Could you check a few things on this model? Use its own coordinates, in mm. Face numbers are marked on the shaded views. Give positions to 0.01 mm unless a question says otherwise; leave off trailing zeros. Write each loop counter-clockwise with the first axis right and the second up, starting at its lowest first coordinate (ties: lowest second). Pieces come first, ordered by that corner, then holes. Notation, with made-up numbers: (79.5, -35) - (116.5, -35) arc R30 ccw to (116.5, 2) - close; hole circle Ø2 at (-18, 46). An arc over 180 degrees is marked (long way). Answer in a Markdown table with one row per item.
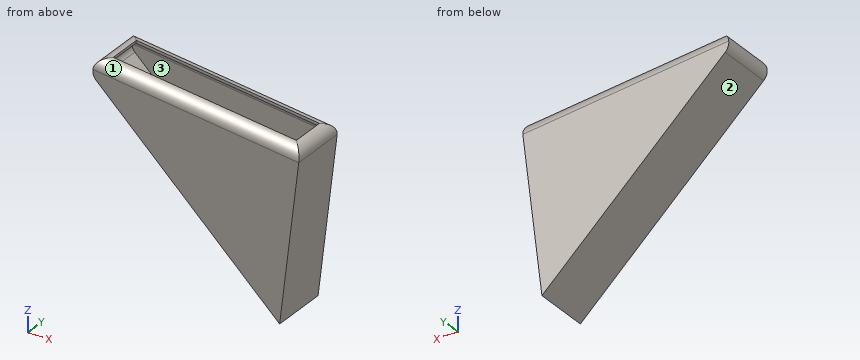
from build123d import *

# Parameters (mm, degrees)
F1_DEPTH = 25.4
F2_R     = 5.08
F3_T     = -1.27


# Not quite as in the source:
# - a shell that OpenCascade refuses in one call is made with other operations: the cavity is built on its own and cut out


with BuildPart() as f1:
    # F0 (on Front) → F1 (new body)
    with BuildSketch(Plane.XZ):
        Polygon((-9.891229794, 75.6632118021), (-110.7755121968, 87.7015490657), (-18.9199827418, 0), align=None)
    extrude(amount=-F1_DEPTH)

    # F2
    f2_edges = [f1.edges().sort_by_distance(p)[0] for p in [
        (-60.333371, 0, 81.68238),
        (-110.775512, 12.7, 87.701549),
        (-60.333371, 25.4, 81.68238),
        (-9.89123, 12.7, 75.663212),
    ]]
    fillet(f2_edges, radius=F2_R)

    # F3: a shell. OpenCascade refuses it in one call, so the cavity is built on its own and cut out:
    # the body offset inwards by the wall thickness, plus a prism from it out through each open face.
    f3_core = offset(f1.part, amount=F3_T, mode=Mode.PRIVATE)
    f3_exits = [f3_core.faces().sort_by_distance(p)[0] for p in [
        (-55.439636, 12.7, 79.81941),
    ]]
    add(f3_core, mode=Mode.SUBTRACT)
    extrude(f3_exits, amount=-F3_T, mode=Mode.SUBTRACT)


solid = f1.part
1) Imagine slicing it at C-C (z = 63). List the corners of the cut face in (x, y) for me.
Check values:
| item | result |
|---|---|
| outline | (-84.9, 0) - (-11.4, 0) - (-11.4, 25.4) - (-84.9, 25.4) - close; hole (-83.06, 1.27) - (-12.68, 1.27) - (-12.68, 24.13) - (-83.06, 24.13) - close |
2) Imagine slicing it at A-A (y = 9). List the corners of the cut face in (x, z) for me, then the cut area to 3 significant figures.
Check values:
| item | result |
|---|---|
| outline | (-99.75, 77.18) - (-18.92, 0) - (-10.49, 70.62) arc R5.08 ccw to (-14.94, 76.27) - (-15.09, 75) arc R3.81 cw to (-11.75, 70.77) - (-19.88, 2.67) - (-98.88, 78.1) arc R3.81 cw to (-95.79, 84.63) - (-95.64, 85.9) arc R5.08 ccw to start |
| area | 252 mm2 |
3) Will these pins go through, and if not, where does the flat tip stop? P1, Ø1.5, axis at x = -72, y = 8.5, coming from the -Z side; P2, Ø5, axis at x = -22, y = 20, coming from the -Z side; P3, Ø23.5, axis at x = -71.5, z = 33.5, coming from the +Y side; P4, Ø6, axis at x = -50.5, y = 12.5, coming from the +Z side.
Check values:
| item | result |
|---|---|
| P1 | stops at z = 49.96 |
| P2 | stops at z = 0.55 |
| P3 | passes through |
| P4 | stops at z = 34.77 |
4) If I drill on line 1 (Y direction, x = -90, z = 76.5); line 2 (X direction, y = 13, z = 81); line 3 (X direction, y = 23.5, z = 16), over which ranges is the centre line in solid material (lowest first)?
Check values:
| item | result |
|---|---|
| line 1 | y = 0 to 1.27, 24.13 to 25.4 |
| line 2 | x = -101.32 to -100.05 |
| line 3 | x = -35.68 to -33.84, -18.29 to -17.01 |
5) Imagine slicing it at B-B (z = 22). List the corners of the cut face in (x, y) for me, then the cut area to 3 significant figures.
Check values:
| item | result |
|---|---|
| outline | (-41.96, 0) - (-16.29, 0) - (-16.29, 25.4) - (-41.96, 25.4) - close; hole (-40.12, 1.27) - (-17.57, 1.27) - (-17.57, 24.13) - (-40.12, 24.13) - close |
| area | 136 mm2 |
6) We'd pull the mould along Z, two halves only. Please class the marked faces 1, 2 and 3: +Z half, -Z half, draft (parallel to the pull), parting line (faces both ways), or undercut.
Check values:
| item | result |
|---|---|
| face 1 | +Z half |
| face 2 | -Z half |
| face 3 | undercut |
